```python
from build123d import *

# Parameters (mm, degrees)
SKETCH1_W               = 90
SKETCH1_H               = 2.5
CUT_EXTRUDE1_DEPTH      = 91.069417673
CUT_EXTRUDE1_DEPTH_BACK = 91.069417673
SKETCH2_W               = 9
SKETCH2_H               = 1
CHAMFER1_SIZE           = 0.2


with BuildPart() as part:
    # Sketch1 → Revolve1 (revolve)
    with BuildSketch(Plane(origin=(0, 0, 0), x_dir=(1, 0, 0), z_dir=(0, 1, 0))):
        with Locations((-45, 1.25)):
            Rectangle(SKETCH1_W, SKETCH1_H)
    revolve(axis=Axis((0, 0, 0), (-1, 0, 0)))

    # Sketch2 → Cut-Extrude1 (cut, two sides: drawn at the far end of the back side and taken through both)
    with BuildSketch(Plane(origin=(0, 0, 0), x_dir=(1, 0, 0), z_dir=(0, 1, 0)).offset(-CUT_EXTRUDE1_DEPTH_BACK)):
        with Locations((-4.5, 2)):
            Rectangle(SKETCH2_W, SKETCH2_H)
    extrude(amount=CUT_EXTRUDE1_DEPTH + CUT_EXTRUDE1_DEPTH_BACK, mode=Mode.SUBTRACT)

    # Chamfer1
    chamfer1_edges = [part.edges().sort_by_distance(p)[0] for p in [
        (-90, 0, 2.5),
        (0, 0, 2.5),
    ]]
    chamfer(chamfer1_edges, length=CHAMFER1_SIZE)


solid = part.part
```
Verification items for the finished model (mm, model axes). A direction names the side the tool comes from. Coordinates: 2 decimals unless noted, no trailing zeros. Loops run counter-clockwise (first coordinate to the right, second up) from the corner with the lowest first, then second, coordinate; pieces in that order, holes last. Notation, with made-up numbers: (49.5, 87) - (67.5, 87) arc R25 ccw to (67.5, 115) - close; hole circle Ø9 at (-6, 21.5). An arc over 180 degrees is marked (long way). Put each result on its own line as item: value.
Item 1: Scan lines: line 1 along X through (y, z) = (-1.15, -1.55); line 2 along Y through (x, z) = (-20, 0.25); line 3 along Z through (x, y) = (-37.5, -0.1). Record each from-to range of solid material in increasing order.
Conclusion:
line 1: x = -90 to -9
line 2: y = -2.49 to 2.49
line 3: z = -2.5 to 2.5
Item 2: Gauge pin test, flat ends, axial feed: pin 1 Ø2 at (x, y) = (-32.5, -1.5) entering from +Z; pin 2 Ø1.5 at (x, z) = (-64.5, -1.5) entering from +Y. Record the tip position at first contact, or that the pin passes through.
Conclusion:
pin 1: stops at z = 2.45
pin 2: stops at y = 2.38
Item 3: Section check C-C (x = -22). Enter the section's corners in (y, z).
Conclusion:
outline: circle Ø5 at (0, 0)
Item 4: Set-up check for faces 1 (the face through (-5, 0, -1.5)), 2 (the face through (0, 0, 0)): record each of +Z, -Z, +X, -X, +Y, -Y from which the full face is reachable in a straight line by a thin tool's end or side.
Conclusion:
face 1: -Z, +X, +Y, -Y
face 2: +Z, -Z, +X, +Y, -Y
Item 5: Section check B-B (x = -5.5). Enter the section's corners in (y, z).
Conclusion:
outline: (-2, -1.5) - (2, -1.5) arc R2.5 ccw (long way) to start
Item 6: Section check A-A (y = 0). Enter the section's corners in (x, z).
Conclusion:
outline: (-90, -2.3) - (-89.8, -2.5) - (-9, -2.5) - (-9, -1.5) - (0, -1.5) - (0, 2.3) - (-0.2, 2.5) - (-89.8, 2.5) - (-90, 2.3) - close
